Verification items for this drawing (mm, ordinates from the low corner). A direction names the side the tool comes from. Round coordinates to 2 decimals unless told otherwise and drop trailing zeros. Loops run counter-clockwise (first coordinate to the right, second up) from the corner with the lowest first, then second, coordinate; pieces in that order, holes last. Notation, with made-up numbers: (46, 18.25) - (94, 18.25) arc R14 cw to (94, 39.25) - close; hole circle Ø11 at (-4, -18.5). An arc over 180 degrees is marked (long way). Use a Markdown table: item, result. Add a question column.
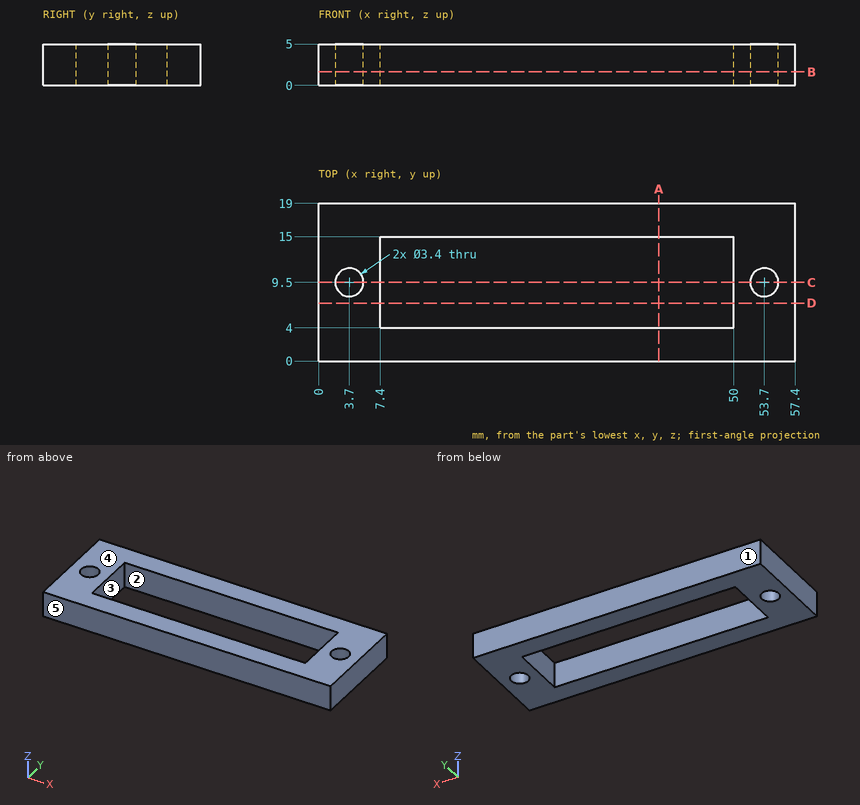
Q1. Section check B-B on z = 1.65. Record the cut outline in (x, y).
Q2. Set-up check for the marked faces 1 and 2: record each of +Z, -Z, +X, -X, +Y, -Y from which the full face is reachable in a straight line by a thin tool's end or side.
Q3. Section check A-A on x = 41. Record the cut outline in (y, z).
Q4. Thickness scan on line 1 along X through (y, z) = (5.5, 2.7); line 2 along Y through (x, z) = (8.5, 1.25); line 3 along Y through (x, z) = (55, 4.7). Record the ranges inside material, lowest first.
Q5. Section check D-D on y = 7. Record the cut outline in (x, z).
Q6. Section check C-C on y = 9.5. Record the cut outline in (x, z), plus the area to 3 significant figures.
Q7. Release check for a two-part mould opening along Y. For the marked faces 3, 4 and 5 record: +Y half, -Y half, draft (parallel to the pull), parting line (faces both ways), or undercut.
Determined:
| question | item | result |
|---|---|---|
| 1 | outline | (0, 0) - (57.4, 0) - (57.4, 19) - (0, 19) - close; hole circle Ø3.4 at (3.7, 9.5); hole (7.4, 4) - (50, 4) - (50, 15) - (7.4, 15) - close; hole circle Ø3.4 at (53.7, 9.5) |
| 2 | face 1 | +Z, -Z, +X, -X, +Y |
| 2 | face 2 | +Z, -Z |
| 3 | outline | (0, 0) - (4, 0) - (4, 5) - (0, 5) - close; (15, 0) - (19, 0) - (19, 5) - (15, 5) - close |
| 4 | line 1 | x = 0 to 7.4, 50 to 57.4 |
| 4 | line 2 | y = 0 to 4, 15 to 19 |
| 4 | line 3 | y = 0 to 8.4, 10.6 to 19 |
| 5 | outline | (0, 0) - (7.4, 0) - (7.4, 5) - (0, 5) - close; (50, 0) - (57.4, 0) - (57.4, 5) - (50, 5) - close |
| 6 | outline | (0, 0) - (2, 0) - (2, 5) - (0, 5) - close; (5.4, 0) - (7.4, 0) - (7.4, 5) - (5.4, 5) - close; (50, 0) - (52, 0) - (52, 5) - (50, 5) - close; (55.4, 0) - (57.4, 0) - (57.4, 5) - (55.4, 5) - close |
| 6 | area | 40.0 mm² |
| 7 | face 3 | undercut |
| 7 | face 4 | draft |
| 7 | face 5 | -Y half |
